from build123d import *

# Parameters (mm, degrees)
SKETCH1_W            = 63.5
SKETCH1_H            = 63.5
SKETCH1_W_2          = 57.15
SKETCH1_H_2          = 57.15
BOSS_EXTRUDE1_DEPTH  = 2.54
SKETCH2_W            = 63.5
SKETCH2_H            = 63.5
BOSS_EXTRUDE2_DEPTH  = 8.89
SKETCH3_R            = 2.54
CUT_EXTRUDE1_DEPTH   = 8.89
SKETCH4_W            = 63.5
SKETCH4_H            = 63.5
SKETCH4_W_2          = 57.15
SKETCH4_H_2          = 57.15
BOSS_EXTRUDE3_DEPTH  = 2.54
SKETCH5_W            = 63.5
SKETCH5_H            = 63.5
BOSS_EXTRUDE4_DEPTH  = 8.89
SKETCH6_R            = 2.54
CUT_EXTRUDE2_DEPTH   = 8.89
SKETCH7_W            = 63.5
SKETCH7_H            = 63.5
SKETCH7_W_2          = 57.15
SKETCH7_H_2          = 57.15
BOSS_EXTRUDE5_DEPTH  = 2.54
SKETCH8_W            = 63.5
SKETCH8_H            = 63.5
BOSS_EXTRUDE6_DEPTH  = 8.89
SKETCH9_R            = 2.54
CUT_EXTRUDE3_DEPTH   = 8.89
SKETCH10_W           = 63.5
SKETCH10_H           = 63.5
SKETCH10_W_2         = 57.15
SKETCH10_H_2         = 57.15
BOSS_EXTRUDE7_DEPTH  = 2.54
SKETCH11_W           = 63.5
SKETCH11_H           = 63.5
BOSS_EXTRUDE8_DEPTH  = 8.89
SKETCH12_R           = 2.54
CUT_EXTRUDE4_DEPTH   = 8.89
SKETCH14_W           = 63.5
SKETCH14_H           = 63.5
SKETCH14_W_2         = 57.15
SKETCH14_H_2         = 57.15
BOSS_EXTRUDE10_DEPTH = 2.54
SKETCH15_W           = 63.5
SKETCH15_H           = 63.5
BOSS_EXTRUDE11_DEPTH = 8.89
SKETCH16_R           = 2.54
CUT_EXTRUDE5_DEPTH   = 8.89
BOSS_EXTRUDE12_REACH = 55.34
SKETCH18_W           = 63.258363329
SKETCH18_H           = 63.5
CUT_EXTRUDE7_REACH   = 53.155
SKETCH19_W           = 21.300485008
SKETCH19_H           = 63.5
BOSS_EXTRUDE15_REACH = 55.34
SKETCH20_W           = 63.5
SKETCH20_H           = 58.16761314
CUT_EXTRUDE8_START   = -13.499985
SKETCH21_W           = 63.5
SKETCH21_H           = 36.305948049
CUT_EXTRUDE8_DEPTH   = 13.499985
BOSS_EXTRUDE16_REACH = 55.34
SKETCH22_W           = 48.076280605
SKETCH22_H           = 63.5
CUT_EXTRUDE9_START   = -0.504151
SKETCH23_W           = 63.5
SKETCH23_H           = 4.915504187
CUT_EXTRUDE9_DEPTH   = 0.504151
BOSS_EXTRUDE18_REACH = 55.34
SKETCH24_W           = 63.5
SKETCH24_H           = 64.511289969
CUT_EXTRUDE10_START  = -26.776858
SKETCH25_W           = 63.5
SKETCH25_H           = 23.443872205
CUT_EXTRUDE10_DEPTH  = 26.776858
SKETCH26_W           = 63.5
SKETCH26_H           = 63.5
BOSS_EXTRUDE19_DEPTH = 41.91


with BuildPart() as part:
    # Sketch1 → Boss-Extrude1 (new body)
    with BuildSketch(Plane(origin=(0, 0, 0), x_dir=(1, 0, 0), z_dir=(0, 1, 0))):
        with Locations((28.575, 28.575)):
            Rectangle(SKETCH1_W, SKETCH1_H)
        with Locations((28.575, 28.575)):
            Rectangle(SKETCH1_W_2, SKETCH1_H_2, mode=Mode.SUBTRACT)
    extrude(amount=BOSS_EXTRUDE1_DEPTH)

    # Sketch2 → Boss-Extrude2 (add)
    with BuildSketch(Plane.XZ):
        with Locations((28.575, -28.575)):
            Rectangle(SKETCH2_W, SKETCH2_H)
    extrude(amount=BOSS_EXTRUDE2_DEPTH)

    # Sketch3 → Cut-Extrude1 (cut)
    with BuildSketch(Plane(origin=(0, 0, 0), x_dir=(1, 0, 0), z_dir=(0, 1, 0))):
        with Locations((28.575, 28.575)):
            Circle(SKETCH3_R)
    extrude(amount=-CUT_EXTRUDE1_DEPTH, mode=Mode.SUBTRACT)



with BuildPart() as body_2:
    # Sketch4 → Boss-Extrude3 (new body)
    with BuildSketch(Plane(origin=(0.678769335, 7.758369005, 0), x_dir=(0, 0, -1), z_dir=(0.087155743, 0.996194698, 0))):
        with Locations((28.575, -91.624069576)):
            Rectangle(SKETCH4_W, SKETCH4_H)
        with Locations((28.575, -91.624069576)):
            Rectangle(SKETCH4_W_2, SKETCH4_H_2, mode=Mode.SUBTRACT)
    extrude(amount=-BOSS_EXTRUDE3_DEPTH)

    # Sketch5 → Boss-Extrude4 (add)
    with BuildSketch(Plane(origin=(0.457393749, 5.228034472, 0), x_dir=(0.996194698, -0.087155743, 0), z_dir=(-0.087155743, -0.996194698, 0))):
        with Locations((91.624069576, -28.575)):
            Rectangle(SKETCH5_W, SKETCH5_H)
    extrude(amount=BOSS_EXTRUDE4_DEPTH)

    # Sketch6 → Cut-Extrude2 (cut)
    with BuildSketch(Plane(origin=(0.457393749, 5.228034472, 0), x_dir=(0.996194698, -0.087155743, 0), z_dir=(0.087155743, 0.996194698, 0))):
        with Locations((91.624069576, 28.575)):
            Circle(SKETCH6_R)
    extrude(amount=-CUT_EXTRUDE2_DEPTH, mode=Mode.SUBTRACT)


with BuildPart() as part_1:
    add(part.part)

    add(body_2.part)  # Boss-Extrude5 merges body 2
    # Sketch7 → Boss-Extrude5 (add)
    with BuildSketch(Plane(origin=(0, 17.451102263, -4.676008758), x_dir=(-1, 0, 0), z_dir=(0, 0.965925826, -0.258819045))):
        with Locations((-28.575, -89.362075096)):
            Rectangle(SKETCH7_W, SKETCH7_H)
        with Locations((-28.575, -89.362075096)):
            Rectangle(SKETCH7_W_2, SKETCH7_H_2, mode=Mode.SUBTRACT)
    extrude(amount=-BOSS_EXTRUDE5_DEPTH)

    # Sketch8 → Boss-Extrude6 (add)
    with BuildSketch(Plane(origin=(0, 14.997650664, -4.018608384), x_dir=(1, 0, 0), z_dir=(0, -0.965925826, 0.258819045))):
        with Locations((28.575, -89.362075096)):
            Rectangle(SKETCH8_W, SKETCH8_H)
    extrude(amount=BOSS_EXTRUDE6_DEPTH)

    # Sketch9 → Cut-Extrude3 (cut)
    with BuildSketch(Plane(origin=(0, 14.997650664, -4.018608384), x_dir=(1, 0, 0), z_dir=(0, 0.965925826, -0.258819045))):
        with Locations((28.575, 89.362075096)):
            Circle(SKETCH9_R)
    extrude(amount=-CUT_EXTRUDE3_DEPTH, mode=Mode.SUBTRACT)

    # Sketch10 → Boss-Extrude7 (add)
    with BuildSketch(Plane(origin=(0, 3.279815329, 1.893602263), x_dir=(1, 0, 0), z_dir=(0, 0.866025404, 0.5))):
        with Locations((28.575, -33.229630657)):
            Rectangle(SKETCH10_W, SKETCH10_H)
        with Locations((28.575, -33.229630657)):
            Rectangle(SKETCH10_W_2, SKETCH10_H_2, mode=Mode.SUBTRACT)
    extrude(amount=-BOSS_EXTRUDE7_DEPTH)

    # Sketch11 → Boss-Extrude8 (add)
    with BuildSketch(Plane(origin=(0, 1.080110803, 0.623602263), x_dir=(1, 0, 0), z_dir=(0, -0.866025404, -0.5))):
        with Locations((28.575, 33.229630657)):
            Rectangle(SKETCH11_W, SKETCH11_H)
    extrude(amount=BOSS_EXTRUDE8_DEPTH)

    # Sketch12 → Cut-Extrude4 (cut)
    with BuildSketch(Plane(origin=(0, 1.080110803, 0.623602263), x_dir=(1, 0, 0), z_dir=(0, 0.866025404, 0.5))):
        with Locations((28.575, -33.229630657)):
            Circle(SKETCH12_R)
    extrude(amount=-CUT_EXTRUDE4_DEPTH, mode=Mode.SUBTRACT)

    # Sketch14 → Boss-Extrude10 (add)
    with BuildSketch(Plane(origin=(-2.8575, 2.8575, 0), x_dir=(0, 0, 1), z_dir=(-0.707106781, 0.707106781, 0))):
        with Locations((-28.575, -32.199012806)):
            Rectangle(SKETCH14_W, SKETCH14_H)
        with Locations((-28.575, -32.199012806)):
            Rectangle(SKETCH14_W_2, SKETCH14_H_2, mode=Mode.SUBTRACT)
    extrude(amount=-BOSS_EXTRUDE10_DEPTH)

    # Sketch15 → Boss-Extrude11 (add)
    with BuildSketch(Plane(origin=(-1.061448776, 1.061448776, 0), x_dir=(0, 0, -1), z_dir=(0.707106781, -0.707106781, 0))):
        with Locations((28.575, -32.199012806)):
            Rectangle(SKETCH15_W, SKETCH15_H)
    extrude(amount=BOSS_EXTRUDE11_DEPTH)

    # Sketch16 → Cut-Extrude5 (cut)
    with BuildSketch(Plane(origin=(-1.061448776, 1.061448776, 0), x_dir=(0, 0, 1), z_dir=(-0.707106781, 0.707106781, 0))):
        with Locations((-28.575, -32.199012806)):
            Circle(SKETCH16_R)
    extrude(amount=-CUT_EXTRUDE5_DEPTH, mode=Mode.SUBTRACT)

    # Boss-Extrude12: up to this face of the body (flat: up to its plane)
    boss_extrude12_end = Plane(part_1.part.faces().sort_by_distance((60.351110962, -8.935945156, -58.051047878))[0])
    # Sketch18 → Boss-Extrude12 (add, up to the picked face)
    with BuildSketch(Plane(origin=(0, -50.8, 0), x_dir=(1, 0, 0), z_dir=(0, 1, 0)), mode=Mode.PRIVATE) as boss_extrude12_sk1:
        with Locations((91.954181664, 28.575)):
            Rectangle(SKETCH18_W, SKETCH18_H)
    boss_extrude12_tool1 = split(extrude(boss_extrude12_sk1.sketch, amount=BOSS_EXTRUDE12_REACH, mode=Mode.PRIVATE), bisect_by=boss_extrude12_end, keep=Keep.BOTH, mode=Mode.PRIVATE)
    add(boss_extrude12_tool1.solids().sort_by_distance((91.954182, -50.8, -28.575))[0])

    # Cut-Extrude7: up to this face of the body (flat: up to its plane)
    cut_extrude7_end = Plane(part_1.part.faces().sort_by_distance((91.954181664, -50.8, -28.575))[0])
    # Sketch19 → Cut-Extrude7 (cut, up to the picked face)
    with BuildSketch(Plane(origin=(-0.317420804, -3.628136394, 0), x_dir=(0.996194698, -0.087155743, 0), z_dir=(0.087155743, 0.996194698, 0)), mode=Mode.PRIVATE) as cut_extrude7_sk1:
        with Locations((134.02431208, 28.575)):
            Rectangle(SKETCH19_W, SKETCH19_H)
    cut_extrude7_tool1 = split(extrude(cut_extrude7_sk1.sketch, amount=-CUT_EXTRUDE7_REACH, mode=Mode.PRIVATE), bisect_by=cut_extrude7_end, keep=Keep.BOTH, mode=Mode.PRIVATE)
    add(cut_extrude7_tool1.solids().sort_by_distance((133.196888, -15.309125, -28.575))[0], mode=Mode.SUBTRACT)

    # Boss-Extrude15: up to this face of the body (flat: up to its plane)
    boss_extrude15_end = Plane(part_1.part.faces().sort_by_distance((-1.691883068, -11.096545593, 3.934189806))[0])
    # Sketch20 → Boss-Extrude15 (add, up to the picked face)
    with BuildSketch(Plane(origin=(0, -50.8, 0), x_dir=(1, 0, 0), z_dir=(0, 1, 0)), mode=Mode.PRIVATE) as boss_extrude15_sk1:
        with Locations((28.575, -29.08380657)):
            Rectangle(SKETCH20_W, SKETCH20_H)
    boss_extrude15_tool1 = split(extrude(boss_extrude15_sk1.sketch, amount=BOSS_EXTRUDE15_REACH, mode=Mode.PRIVATE), bisect_by=boss_extrude15_end, keep=Keep.BOTH, mode=Mode.PRIVATE)
    add(boss_extrude15_tool1.solids().sort_by_distance((28.575, -50.8, 29.083807))[0])

    # Sketch21 → Cut-Extrude8 (cut)
    with BuildSketch(Plane(origin=(0, -6.618855037, -3.821397737), x_dir=(1, 0, 0), z_dir=(0, 0.866025404, 0.5)).offset(CUT_EXTRUDE8_START)):
        with Locations((28.575, -83.132604681)):
            Rectangle(SKETCH21_W, SKETCH21_H)
    extrude(amount=CUT_EXTRUDE8_DEPTH, mode=Mode.SUBTRACT)

    # Boss-Extrude16: up to this face of the body (flat: up to its plane)
    boss_extrude16_end = Plane(part_1.part.faces().sort_by_distance((-3.786785852, -14.23624687, 1.5875))[0])
    # Sketch22 → Boss-Extrude16 (add, up to the picked face)
    with BuildSketch(Plane(origin=(0, -50.8, 0), x_dir=(1, 0, 0), z_dir=(0, 1, 0)), mode=Mode.PRIVATE) as boss_extrude16_sk1:
        with Locations((-24.038140303, 28.575)):
            Rectangle(SKETCH22_W, SKETCH22_H)
    boss_extrude16_tool1 = split(extrude(boss_extrude16_sk1.sketch, amount=BOSS_EXTRUDE16_REACH, mode=Mode.PRIVATE), bisect_by=boss_extrude16_end, keep=Keep.BOTH, mode=Mode.PRIVATE)
    add(boss_extrude16_tool1.solids().sort_by_distance((-24.03814, -50.8, -28.575))[0])

    # Sketch23 → Cut-Extrude9 (cut)
    with BuildSketch(Plane(origin=(5.224730509, -5.224730509, 0), x_dir=(0, 0, 1), z_dir=(-0.707106781, 0.707106781, 0)).offset(CUT_EXTRUDE9_START)):
        with Locations((-28.575, -66.4067649)):
            Rectangle(SKETCH23_W, SKETCH23_H)
    extrude(amount=CUT_EXTRUDE9_DEPTH, mode=Mode.SUBTRACT)

    # Boss-Extrude18: up to this face of the body (flat: up to its plane)
    boss_extrude18_end = Plane(part_1.part.faces().sort_by_distance((-1.009372862, -9.522895431, -61.182209856))[0])
    # Sketch24 → Boss-Extrude18 (add, up to the picked face)
    with BuildSketch(Plane(origin=(0, -50.8, 0), x_dir=(1, 0, 0), z_dir=(0, 1, 0)), mode=Mode.PRIVATE) as boss_extrude18_sk1:
        with Locations((28.575, 89.405644985)):
            Rectangle(SKETCH24_W, SKETCH24_H)
    boss_extrude18_tool1 = split(extrude(boss_extrude18_sk1.sketch, amount=BOSS_EXTRUDE18_REACH, mode=Mode.PRIVATE), bisect_by=boss_extrude18_end, keep=Keep.BOTH, mode=Mode.PRIVATE)
    add(boss_extrude18_tool1.solids().sort_by_distance((28.575, -50.8, -89.405645))[0])

    # Sketch25 → Cut-Extrude10 (cut)
    with BuildSketch(Plane(origin=(0, 6.410570068, -1.717707073), x_dir=(1, 0, 0), z_dir=(0, 0.965925826, -0.258819045)).offset(CUT_EXTRUDE10_START)):
        with Locations((28.575, 132.834011199)):
            Rectangle(SKETCH25_W, SKETCH25_H)
    extrude(amount=CUT_EXTRUDE10_DEPTH, mode=Mode.SUBTRACT)

    # Sketch26 → Boss-Extrude19 (add)
    with BuildSketch(Plane(origin=(0, -50.8, 0), x_dir=(1, 0, 0), z_dir=(0, 1, 0))):
        with Locations((28.575, 28.575)):
            Rectangle(SKETCH26_W, SKETCH26_H)
    extrude(amount=BOSS_EXTRUDE19_DEPTH)


solid = part_1.part
Source: CAD feature listing. Evaluate the final solid. Frame: model axes, mm. A direction names the side the tool comes from. Round coordinates to 2 decimals unless told otherwise and drop trailing zeros. Loops run counter-clockwise (first coordinate to the right, second up) from the corner with the lowest first, then second, coordinate; pieces in that order, holes last. Notation, with made-up numbers: (29, 71) -> (35, 71) arc R18 cw to (35, 100) -> close; hole circle Ø3 at (-27, 56). An arc over 180 degrees is marked (long way). Answer as a JSON object with one key per item and string values. Group by question number.
Q1. Contact query for flat-ended pins moving along their axis: P1, Ø4, axis at x = -18.5, z = -62.5, coming from the -Y side; P2, Ø10, axis at x = -23.5, y = -14, coming from the -Z side (3 decimals); P3, Ø10, axis at y = -24, z = -27.5, coming from the +X side; P4, Ø3, axis at x = 36, y = 1, coming from the +Z side. Output: stop coordinate, or through.
Q2. Mould query, pull axis Y, two halves, no side actions, for faces 1 (the flat face through (92, -25, 3.175)), 2 (the flat face through (121.52, -26.56, -28.13)), 3 (the flat face through (28.54, -16.71, -88)). Classes: pulls with the +Y half, pulls with the -Y half, needs draft (parallel to the pull), parting line crosses it, or undercut.
Q3. Ray query, line 1 (Z direction, x = -31, y = -28) (3 decimals); line 2 (X direction, y = -13.5, z = 27) (3 decimals); line 3 (Z direction, x = 82.5, y = -33) (3 decimals). Return the intervals inside material, ascending. Write a range as from..to.
Q4. Section query A-A (z = -45). Output: boundary loops of the cut face in (x, y) (3 decimals), plus the area to 3 significant figures.
Q5. Section query D-D (x = 109). Output: boundary loops of the cut face in (y, z) (3 decimals).
Q6. Section query C-C (y = -34). Output: boundary loops of the cut face in (x, z) (3 decimals).
Q7. Access query for faces 4 (the flat face through (-3.175, -30, 25)), 5 (the cylindrical face through (26.037, -19.274, 27.113)), 6 (the flat face through (92, -2, 0)). Directions: +Z, -Z, +X, -X, +Y, -Y. A direction counts if a zero-diameter tool reaches every point of the face in a straight line with its end or side. Return the directions, or none.
Completed:
{
 "1": {"P1": "through", "P2": "z = -60.325", "P3": "x = 122.18", "P4": "z = 5.92"},
 "2": {"face 1": "needs draft", "face 2": "pulls with the -Y half", "face 3": "undercut"},
 "3": {"line 1": "-60.325..-57.15, 0..3.175", "line 2": "-3.175..0, 57.15..60.325", "line 3": "-60.325..3.175"},
 "4": {"outline": "(-48.076, -42.361) -> (-39.638, -50.8) -> (119.401, -50.8) -> (123.583, -2.994) -> (120.42, -2.718) -> (120.199, -5.248) -> (63.267, -0.267) -> (63.488, 2.263) -> (60.325, 2.54) -> (57.15, 2.54) -> (57.15, 0) -> (0, 0) -> (0, 2.54) -> (-3.175, 2.54) -> (-5.42, 0.295) -> (-3.624, -1.501) -> (-44.035, -41.912) -> (-45.831, -40.116) -> close", "area": "7,400 mm²"},
 "5": {"outline": "(-50.8, -60.325) -> (-1.719, -60.325) -> (-1.719, -57.15) -> (-4.268, -57.15) -> (-4.268, 0) -> (-1.719, 0) -> (-1.719, 3.175) -> (-50.8, 3.175) -> close"},
 "6": {"outline": "(-39.715, -60.325) -> (-3.175, -60.325) -> (-3.175, -116.274) -> (60.325, -116.274) -> (60.325, -60.325) -> (120.871, -60.325) -> (120.871, 3.175) -> (60.325, 3.175) -> (60.325, 55.402) -> (-3.175, 55.402) -> (-3.175, 3.175) -> (-39.715, 3.175) -> (-39.715, 0) -> (-36.123, 0) -> (-36.123, -57.15) -> (-39.715, -57.15) -> close"},
 "7": {"face 4": "+Z, -X, +Y, -Y", "face 5": "none", "face 6": "+Y"}
}
